Could you check a few things on this model? Use its own coordinates, in mm. Face numbers are marked on the shaded views. A direction names the side the tool comes from. Give positions to 0.01 mm unless a question says otherwise; leave off trailing zeros. Write each loop counter-clockwise with the first axis right and the second up, starting at its lowest first coordinate (ties: lowest second). Pieces come first, ordered by that corner, then holes. Notation, with made-up numbers: M -1,83 L 28,83 A23 cw 28,100 Z; hole C 87.25,20 d11. An arc over 180 degrees is marked long. One line per item, written item: value.
```python
from build123d import *

# Parameters (mm, degrees)
SKETCH1_R           = 0.5
SKETCH1_R_2         = 0.75
SKETCH1_R_3         = 1
BOSS_EXTRUDE1_DEPTH = 2
SKETCH2_R           = 1.75
SKETCH2_R_2         = 1.25
EXTRUDE_THIN1_DEPTH = 2


with BuildPart() as part:
    # Sketch1 → Boss-Extrude1 (new body)
    with BuildSketch(Plane(origin=(0, 0, 0), x_dir=(1, 0, 0), z_dir=(0, 1, 0))):
        with BuildLine():
            Line((-4.710957819, 1.675373519), (-0.920020296, 12.335054222))
            ThreePointArc((-0.920020296, 12.335054222), (0.024018874, 12.999977811), (0.965594569, 12.331570343))
            Line((0.965594569, 12.331570343), (4.717116505, 1.657954125))
            ThreePointArc((4.717116505, 1.657954125), (5, 0), (4.717116505, -1.657954125))
            Line((4.717116505, -1.657954125), (0.965594569, -12.331570343))
            ThreePointArc((0.965594569, -12.331570343), (0.024018874, -12.999977811), (-0.920020296, -12.335054222))
            Line((-0.920020296, -12.335054222), (-4.710957819, -1.675373519))
            ThreePointArc((-4.710957819, -1.675373519), (-5, 0), (-4.710957819, 1.675373519))
        make_face()
        with Locations(Location((0.022171268, 9.122391825, 0), (0, 0, 270))):
            Circle(SKETCH1_R, mode=Mode.SUBTRACT)
        with Locations(Location((0.022171268, 6.764981493, 0), (0, 0, 270))):
            Circle(SKETCH1_R_2, mode=Mode.SUBTRACT)
        with Locations(Location((0.022171268, 3.000162006, 0), (0, 0, 270))):
            Circle(SKETCH1_R_3, mode=Mode.SUBTRACT)
        with Locations(Location((0.022171268, -9.122391825, 0), (0, 0, 90))):
            Circle(SKETCH1_R, mode=Mode.SUBTRACT)
        with Locations(Location((0.022171268, -6.764981493, 0), (0, 0, 90))):
            Circle(SKETCH1_R_2, mode=Mode.SUBTRACT)
        with Locations(Location((0.022171268, -3.000162006, 0), (0, 0, 90))):
            Circle(SKETCH1_R_3, mode=Mode.SUBTRACT)
    extrude(amount=BOSS_EXTRUDE1_DEPTH)

    # Sketch2 → Extrude-Thin1 (add)
    with BuildSketch(Plane(origin=(0, 2, 0), x_dir=(1, 0, 0), z_dir=(0, 1, 0))):
        Circle(SKETCH2_R)
        Circle(SKETCH2_R_2, mode=Mode.SUBTRACT)
    extrude(amount=EXTRUDE_THIN1_DEPTH)


solid = part.part
```
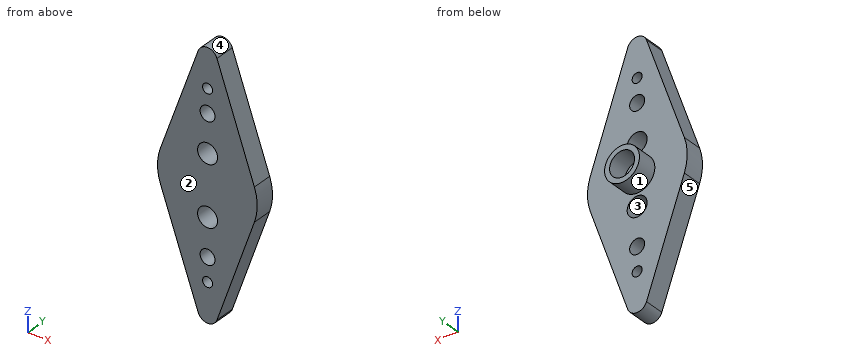
1) If we section it at D-D, the plane x = -3.75: Write out the boundary of the cut face in (y, z).
Outcome:
outline: M 0,-4.38 L 2,-4.38 L 2,4.38 L 0,4.38 Z
2) If we section it at A-A, the plane z = 0: Write out the boundary of the cut face in (x, y).
Outcome:
outline: M -5,0 L 5,0 L 5,2 L 1.75,2 L 1.75,4 L 1.25,4 L 1.25,2 L -1.25,2 L -1.25,4 L -1.75,4 L -1.75,2 L -5,2 Z
3) If we section it at C-C, the plane x = -0.25: Give the number of separate pieces and of enclosed holes in the cut face, then the cut area to 3 significant figures.
Outcome:
separate pieces: 7
enclosed holes: 0
area: 37.2 mm^2
4) On a 3-axis mill with a long thin cutter (end or side, diameter ignored), from which of +Z, -Z, +X, -X, +Y, -Y can I reach the whole of each face in a straight line? I mean the marked faces 1 and 2. Say none if no direction works.
Outcome:
face 1: +Y
face 2: +Z, -Z, +X, -X, -Y
5) I'm going to push flat-ended pins straight in: pin 1 (1.4 mm diameter, centred on x = 0.02, z = 6.76, fed in from +Y); pin 2 (1 mm diameter, centred on y = 2, z = -4, fed in from +X). Where does each tip first touch, or does it pass through?
Outcome:
pin 1: passes through
pin 2: stops at x = 4.07
6) Please list where these lines run through material, in increasing order: L1, parallel to Z at x = 0, y = 3.35; L2, parallel to Y at x = 0, z = -4.75; L3, parallel to X at y = 1, z = 0.75. Write a range as from..to.
Outcome:
L1: z = -1.75..-1.25, 1.25..1.75
L2: y = 0..2
L3: x = -4.94..4.94
7) If we section it at B-B, the plane y = 1.7: Write out the boundary of the cut face in (x, z).
Outcome:
outline: M -4.71,-1.68 L -0.92,-12.34 A1 ccw 0.97,-12.33 L 4.72,-1.66 A5 ccw 4.72,1.66 L 0.97,12.33 A1 ccw -0.92,12.34 L -4.71,1.68 A5 ccw Z; hole C 0.02,-3 d2; hole C 0.02,3 d2; hole C 0.02,-6.76 d1.5; hole C 0.02,6.76 d1.5; hole C 0.02,-9.12 d1; hole C 0.02,9.12 d1
8) We'd pull the mould along X, two halves only. Please class the marked faces 3, 4 and 5: pulls with the +X half, pulls with the -X half, needs draft (parallel to the pull), parting line crosses it, or undercut.
Outcome:
face 3: undercut
face 4: parting line crosses it
face 5: pulls with the -X half
